from build123d import *

# Parameters (mm, degrees)
SKETCH1_R           = 1.8
BOSS_EXTRUDE1_DEPTH = 12.28
CUT_EXTRUDE1_DEPTH  = 6
SKETCH1_4_R         = 1.8
CUT_EXTRUDE2_DEPTH  = 8
SKETCH2_W           = 8
SKETCH2_H           = 9
SKETCH2_R           = 1.4
BOSS_EXTRUDE2_DEPTH = 3
FILLET1_R           = 1
CHAMFER1_SIZE       = 0.5


with BuildPart() as part:
    # Sketch1 → Boss-Extrude1 (new body)
    # profile 1 of 5: a face of its own
    with BuildSketch(Plane.XY):
        Polygon((36, 28.4), (25.4, 28.4), (25.4, 27.4), (25.4, 20.4), (25.4, 19.4), (36, 19.4), align=None)
        with Locations((32, 23.9)):
            Circle(SKETCH1_R, mode=Mode.SUBTRACT)
    # profile 2 of 5: a face of its own
    with BuildSketch(Plane.XY):
        with Locations((32, 23.9)):
            Circle(SKETCH1_R)
    # profile 3 of 5: a face of its own
    with BuildSketch(Plane.XY):
        Polygon((-12.94, 28.4), (-36, 28.4), (-36, 19.4), (-12.94, 19.4), (-12.94, 20.4), (-12.94, 27.4), align=None)
        with Locations((-32, 23.9)):
            Circle(SKETCH1_R, mode=Mode.SUBTRACT)
    # profile 4 of 5: a face of its own
    with BuildSketch(Plane.XY):
        with Locations((-32, 23.9)):
            Circle(SKETCH1_R)
    # profile 5 of 5: a face of its own
    with BuildSketch(Plane.XY):
        Polygon((25.4, 28.4), (-12.94, 28.4), (-12.94, 27.4), (-12.94, 20.4), (-12.94, 19.4), (25.4, 19.4), (25.4, 20.4), (25.4, 27.4), align=None)
    extrude(amount=BOSS_EXTRUDE1_DEPTH)

    # Sketch1<3> → Cut-Extrude1 (cut)
    with BuildSketch(Plane.XY):
        Polygon((25.4, 28.4), (-12.94, 28.4), (-12.94, 27.4), (-12.94, 20.4), (-12.94, 19.4), (25.4, 19.4), (25.4, 20.4), (25.4, 27.4), align=None)
    extrude(amount=CUT_EXTRUDE1_DEPTH, mode=Mode.SUBTRACT)

    # Sketch1<4> → Cut-Extrude2 (cut)
    with BuildSketch(Plane.XY):
        with Locations((-32, 23.9)):
            Circle(SKETCH1_4_R)
        with Locations((32, 23.9)):
            Circle(SKETCH1_4_R)
    extrude(amount=CUT_EXTRUDE2_DEPTH, mode=Mode.SUBTRACT)

    # Sketch2 → Boss-Extrude2 (add)
    # profile 1 of 2: a face of its own
    with BuildSketch(Plane.XY.offset(12.28)):
        with Locations((-40, 23.9)):
            Rectangle(SKETCH2_W, SKETCH2_H)
        with Locations((-40, 23.9)):
            Circle(SKETCH2_R, mode=Mode.SUBTRACT)
    # profile 2 of 2: a face of its own
    with BuildSketch(Plane.XY.offset(12.28)):
        with Locations((40, 23.9)):
            Rectangle(SKETCH2_W, SKETCH2_H)
        with Locations((40, 23.9)):
            Circle(SKETCH2_R, mode=Mode.SUBTRACT)
    extrude(amount=-BOSS_EXTRUDE2_DEPTH)

    # Fillet1
    fillet1_edges = [part.edges().sort_by_distance(p)[0] for p in [
        (-12.94, 19.4, 3),
        (25.4, 19.4, 3),
        (25.4, 28.4, 3),
        (-12.94, 28.4, 3),
        (-36, 28.4, 4.64),
        (-36, 19.4, 4.64),
        (36, 28.4, 4.64),
        (36, 19.4, 4.64),
        (-44, 19.4, 10.78),
        (-44, 28.4, 10.78),
        (44, 19.4, 10.78),
        (44, 28.4, 10.78),
    ]]
    fillet(fillet1_edges, radius=FILLET1_R)

    # Chamfer1
    chamfer1_edges = [part.edges().sort_by_distance(p)[0] for p in [
        (-33.8, 23.9, 0),
        (30.2, 23.9, 0),
    ]]
    chamfer(chamfer1_edges, length=CHAMFER1_SIZE)


solid = part.part
Here's how the part is built. I have some questions about the finished solid (model axes, mm). A direction names the side the tool comes from. Round coordinates to 2 decimals unless told otherwise and drop trailing zeros. Write each loop counter-clockwise with the first axis right and the second up, starting at its lowest first coordinate (ties: lowest second). Pieces come first, ordered by that corner, then holes.
1. For faces 1 (the flat face through (-36, 24, 5)), 2 (the flat face through (-12.94, 24, 3)), 3 (the flat face through (-44, 24, 11)), 4 (the flat face through (-32, 24, 8)), which set-ups out of +Z, -Z, +X, -X, +Y, -Y let a thin tool reach every point of the face, with its end or its side?
2. Suppose I cut it at B-B (z = 3). List the corners of the cut face in (x, y) for me, and give its area (3 significant figures).
3. Suppose I cut it at C-C (x = 40). List the corners of the cut face in (y, z) for me.
4. Will these pins go through, and if not, where does the flat tip stop? pin 1 Ø4 at (x, y) = (14.5, 24) entering from -Z; pin 2 Ø4.5 at (x, y) = (-41, 23) entering from -Z; pin 3 Ø5 at (y, z) = (23, 2.5) entering from +X; pin 4 Ø1.7 at (x, y) = (40, 23.9) entering from +Z.
5. If we mould it in two halves opening along Y, with no side actions, what happens to faces 5 (the flat face through (36, 24, 5)), 6 (the flat face through (-1, 28.4, 8)), 7 (the cylindrical face through (-30.337, 23.211, 4.198))? For each: released by +Y, released by -Y, zero draft, split by the parting line, or undercut.
6. I need wall thicknesses on L1, parallel to X at y = 21.25, z = 2.25; L2, parallel to Y at x = 32, z = 4; L3, parallel to Y at x = -40, z = 11.45. Which ranges of each line are inside material? Lowest first, please.
7. Suppose I cut it at A-A (y = 23.9). State how many separate pieces and enclosed holes the cut face has, and give its area (3 significant figures).
8. Suppose I cut it at D-D (z = 7.25). List the corners of the cut face in (x, y) for me, and give its area (3 significant figures).
Answer sheet:
1. face 1: -Z, -X, +Y, -Y
1. face 2: -Z, +Y, -Y
1. face 3: +Z, -Z, -X, +Y, -Y
1. face 4: -Z
2. outline: (-36, 20.4) arc R1 ccw to (-35, 19.4) - (-13.94, 19.4) arc R1 ccw to (-12.94, 20.4) - (-12.94, 27.4) arc R1 ccw to (-13.94, 28.4) - (-35, 28.4) arc R1 ccw to (-36, 27.4) - close; (25.4, 20.4) arc R1 ccw to (26.4, 19.4) - (35, 19.4) arc R1 ccw to (36, 20.4) - (36, 27.4) arc R1 ccw to (35, 28.4) - (26.4, 28.4) arc R1 ccw to (25.4, 27.4) - close; hole circle Ø3.6 at (-32, 23.9); hole circle Ø3.6 at (32, 23.9)
2. area: 281 mm2
3. outline: (19.4, 9.28) - (22.5, 9.28) - (22.5, 12.28) - (19.4, 12.28) - close; (25.3, 9.28) - (28.4, 9.28) - (28.4, 12.28) - (25.3, 12.28) - close
4. pin 1: stops at z = 6
4. pin 2: stops at z = 9.28
4. pin 3: stops at x = 36
4. pin 4: passes through
5. face 5: zero draft
5. face 6: released by +Y
5. face 7: undercut
6. L1: x = -36 to -12.94, 25.4 to 36
6. L2: y = 19.4 to 22.1, 25.7 to 28.4
6. L3: y = 19.4 to 22.5, 25.3 to 28.4
7. separate pieces: 3
7. enclosed holes: 0
7. area: 627 mm2
8. outline: (-36, 20.4) arc R1 ccw to (-35, 19.4) - (35, 19.4) arc R1 ccw to (36, 20.4) - (36, 27.4) arc R1 ccw to (35, 28.4) - (-35, 28.4) arc R1 ccw to (-36, 27.4) - close; hole circle Ø3.6 at (-32, 23.9); hole circle Ø3.6 at (32, 23.9)
8. area: 627 mm2
